Could you check a few things on this model? Use its own coordinates, in mm. A direction names the side the tool comes from. Give positions to 0.01 mm unless a question says otherwise; leave off trailing zeros. Order: outer loops, then holes, each group sorted by start corner. A loop starts at its lowest first (then second) coordinate and runs counter-clockwise, first axis right, second up. Notation, with made-up numbers: (27.5, 81) - (41.5, 81) arc R25 cw to (41.5, 108) - close; hole circle Ø3 at (79, 64). An arc over 180 degrees is marked (long way). One line per question, with ' | ' between items. Start each with the question number.
1. Imagine slicing it at C-C (y = 398). Please give me the cut outline in (x, z), and give its area (3 significant figures).
2. Imagine slicing it at A-A (z = -413.5). Please give me the cut outline in (x, y), and give its area (3 significant figures).
3. Which directions (+Z, -Z, +X, -X, +Y, -Y) give clear straight access to the entire face, cutting with the end or side of a thin tool? Please do faces 4 (the flat face through (-221.105, 37.709, -350.622)), 5 (the flat face through (1112, 53, 0)), 6 (the flat face through (1347.387, 37.709, -350.622)), 7 (the flat face through (-447.122, 57.307, 100.533)).
4. I need wall thicknesses on probe 1 along X at (y, z) = (-402.5, -26.5); probe 2 along X at (y, z) = (-162, -341); probe 3 along Z at (x, y) = (254.5, 186.5). Which ranges of each line are inside material? Lowest first, please. Write a range as from..to.
5. Imagine slicing it at B-B (z = 111.5). Please give me the cut outline in (x, y).
6. For P1, Ø2, axis at x = -174.5, y = 85.5, coming from the +Z side; P2, Ø5, axis at x = 191, y = -241.5, coming from the -Z side; P3, Ø3, axis at y = 343, z = -550, coming from the +X side, each with a flat end and sliding along its axis, tell me the tip position at first contact or that it passes through.
7. Imagine slicing it at D-D (x = 145.5). Please give me the cut outline in (y, z).
8. If we mould it in two halves opening along X, with no side actions, what happens to faces 1 (the flat face through (329, -489.316, 13)), 2 (the flat face through (1089.95, 59.11, 100.53)), 3 (the flat face through (880.532, 52.676, -350.622))? For each: released by +X, released by -X, zero draft, split by the parting line, or undercut.
```python
from build123d import *

# Parameters (mm, degrees)
F1_DEPTH = 25.4
F3_DEPTH = 152.4
F5_DEPTH = 711.2


with BuildPart() as f1:
    # F0 (on Top) → F1 (new body)
    with BuildSketch(Plane.XY):
        Polygon((-823.540136, 579.701138), (-599.702636, -489.315987), (1249.734864, -489.315987), (1473.572364, 579.701138), align=None)
    extrude(amount=F1_DEPTH)

    # F2 (on face) → F3 (join)
    with BuildSketch(Plane.XY.offset(25.4)):
        Polygon((1473.572364, 579.701138), (-823.540136, 579.701138), (-700.884281, -6.086362), (-186.153281, 122.501138), (836.196719, 122.501138), (1350.916509, -6.086362), align=None)
    extrude(amount=F3_DEPTH)

    # F4 (on face) → F5 (join)
    with BuildSketch(Plane(origin=(0, 0, 0), x_dir=(1, 0, 0), z_dir=(0, 0, -1))):
        Polygon((-810.840136, -579.701138), (-587.002636, 489.315987), (-599.702636, 489.315987), (-823.540136, -579.701138), align=None)
        Polygon((-321.890136, -579.701138), (-98.052636, 489.315987), (-110.752636, 489.315987), (-334.590136, -579.701138), align=None)
        Polygon((984.622364, -579.701138), (773.484864, 489.315987), (760.784864, 489.315987), (971.922364, -579.701138), align=None)
        Polygon((1473.572364, -579.701138), (1249.734864, 489.315987), (1237.034864, 489.315987), (1460.872364, -579.701138), align=None)
    extrude(amount=F5_DEPTH)


solid = f1.part
```
Results found:
1) outline: (-785.49, -711.2) - (-772.79, -711.2) - (-772.79, 0) - (-296.54, 0) - (-296.54, -711.2) - (-283.84, -711.2) - (-283.84, 0) - (936.04, 0) - (936.04, -711.2) - (948.74, -711.2) - (948.74, 0) - (1422.83, 0) - (1422.83, -711.2) - (1435.53, -711.2) - (1435.53, 177.8) - (-785.49, 177.8) - close | area: 431,000 mm2
2) outline: (-823.54, 579.7) - (-599.7, -489.32) - (-587, -489.32) - (-810.84, 579.7) - close; (-334.59, 579.7) - (-110.75, -489.32) - (-98.05, -489.32) - (-321.89, 579.7) - close; (760.78, -489.32) - (773.48, -489.32) - (984.62, 579.7) - (971.92, 579.7) - close; (1237.03, -489.32) - (1249.73, -489.32) - (1473.57, 579.7) - (1460.87, 579.7) - close | area: 54,300 mm2
3) face 4: -Z, -Y | face 5: -Z | face 6: -Z, +Y | face 7: +Z, -Y
4) probe 1: x = -617.88..-605.18, -128.93..-116.23, 777.93..790.63, 1255.21..1267.91 | probe 2: x = -668.24..-655.54, -179.29..-166.59, 825.43..838.13, 1305.57..1318.27 | probe 3: z = 0..177.8
5) outline: (-823.54, 579.7) - (-700.88, -6.09) - (-186.15, 122.5) - (836.2, 122.5) - (1350.92, -6.09) - (1473.57, 579.7) - close
6) P1: stops at z = 25.4 | P2: stops at z = 0 | P3: stops at x = 1424.32
7) outline: (-489.32, 0) - (579.7, 0) - (579.7, 177.8) - (122.5, 177.8) - (122.5, 25.4) - (-489.32, 25.4) - close
8) face 1: zero draft | face 2: undercut | face 3: undercut
